from build123d import *

# Parameters (mm, degrees)
F0_R     = 1.45
F1_DEPTH = 1.5
F2_DEPTH = 18
F3_R     = 0.9
F4_DEPTH = 5
F6_DEPTH = 5
F7_R     = 3.8


with BuildPart() as f1:
    # F0 (on Top) → F1 (new body)
    with BuildSketch(Plane.XY):
        with BuildLine():
            Line((-2.6044162591, 5.2848328158), (-11.2348561883, 5.2848328158))
            Line((-11.2348561883, 5.2848328158), (-11.2348561883, -6.4651671842))
            Line((-11.2348561883, -6.4651671842), (-2.6044162591, -6.4651671842))
            ThreePointArc((-2.6044162591, -6.4651671842), (-0.1771907831, -2.6229563548), (3.2651438117, -5.5901671842))
            ThreePointArc((3.2651438117, -5.5901671842), (3.2323546411, -6.032501779), (3.1347038825, -6.4651671842))
            Line((3.1347038825, -6.4651671842), (7.3955837409, -6.4651671842))
            ThreePointArc((7.3955837409, -6.4651671842), (7.8542311215, -3.8048100771), (10.2651438117, -2.5901671842))
            Line((10.2651438117, -2.5901671842), (10.2651438117, 1.4098328158))
            ThreePointArc((10.2651438117, 1.4098328158), (7.8542311215, 2.6244757087), (7.3955837409, 5.2848328158))
            Line((7.3955837409, 5.2848328158), (3.1347038825, 5.2848328158))
            ThreePointArc((3.1347038825, 5.2848328158), (3.2323546411, 4.8521674106), (3.2651438117, 4.4098328158))
            ThreePointArc((3.2651438117, 4.4098328158), (-0.1771907831, 1.4426219864), (-2.6044162591, 5.2848328158))
        make_face()
        with Locations((-4.7348561883, -0.5901671842)):
            Circle(F0_R, mode=Mode.SUBTRACT)
        with Locations((5.2651438117, -0.5901671842)):
            Circle(F0_R, mode=Mode.SUBTRACT)
        with BuildLine():
            ThreePointArc((10.2651438117, -2.5901671842), (7.8542311215, -3.8048100771), (7.3955837409, -6.4651671842))
            Line((7.3955837409, -6.4651671842), (9.1089107037, -6.4651671842))
            ThreePointArc((9.1089107037, -6.4651671842), (8.9668275944, -4.9445086057), (10.2651438117, -4.1401671842))
            Line((10.2651438117, -4.1401671842), (10.2651438117, -2.5901671842))
        make_face()
        with BuildLine():
            Line((9.1089107037, 5.2848328158), (7.3955837409, 5.2848328158))
            ThreePointArc((7.3955837409, 5.2848328158), (7.8542311215, 2.6244757087), (10.2651438117, 1.4098328158))
            Line((10.2651438117, 1.4098328158), (10.2651438117, 2.9598328158))
            ThreePointArc((10.2651438117, 2.9598328158), (8.9668275944, 3.7641742373), (9.1089107037, 5.2848328158))
        make_face()
        with BuildLine():
            Line((9.1089107037, -6.4651671842), (7.3955837409, -6.4651671842))
            ThreePointArc((7.3955837409, -6.4651671842), (10.7074784065, -8.5573780136), (13.2651438117, -5.5901671842))
            ThreePointArc((13.2651438117, -5.5901671842), (12.6209876096, -3.7327496221), (10.9651438117, -2.672976755))
            ThreePointArc((10.9651438117, -2.672976755), (10.6175843829, -2.6109415057), (10.2651438117, -2.5901671842))
            Line((10.2651438117, -2.5901671842), (10.2651438117, -4.1401671842))
            ThreePointArc((10.2651438117, -4.1401671842), (11.2904486444, -4.5648623515), (11.7151438117, -5.5901671842))
            ThreePointArc((11.7151438117, -5.5901671842), (10.7266424539, -6.9647649448), (9.1089107037, -6.4651671842))
        make_face()
        with BuildLine():
            ThreePointArc((3.1347038825, 5.2848328158), (0.2651438117, 7.4098328158), (-2.6044162591, 5.2848328158))
            Line((-2.6044162591, 5.2848328158), (-0.8910892963, 5.2848328158))
            ThreePointArc((-0.8910892963, 5.2848328158), (0.2651438117, 5.8598328158), (1.4213769197, 5.2848328158))
            Line((1.4213769197, 5.2848328158), (3.1347038825, 5.2848328158))
        make_face()
        with BuildLine():
            Line((-0.8910892963, 5.2848328158), (-2.6044162591, 5.2848328158))
            ThreePointArc((-2.6044162591, 5.2848328158), (-0.1771907831, 1.4426219864), (3.2651438117, 4.4098328158))
            ThreePointArc((3.2651438117, 4.4098328158), (3.2323546411, 4.8521674106), (3.1347038825, 5.2848328158))
            Line((3.1347038825, 5.2848328158), (1.4213769197, 5.2848328158))
            ThreePointArc((1.4213769197, 5.2848328158), (1.6397415722, 4.8713314579), (1.7151438117, 4.4098328158))
            ThreePointArc((1.7151438117, 4.4098328158), (-0.1963548305, 3.0352350552), (-0.8910892963, 5.2848328158))
        make_face()
        with BuildLine():
            ThreePointArc((13.2651438117, 4.4098328158), (10.7074784065, 7.3770436452), (7.3955837409, 5.2848328158))
            Line((7.3955837409, 5.2848328158), (9.1089107037, 5.2848328158))
            ThreePointArc((9.1089107037, 5.2848328158), (10.7266424539, 5.7844305763), (11.7151438117, 4.4098328158))
            ThreePointArc((11.7151438117, 4.4098328158), (11.2904486444, 3.3845279831), (10.2651438117, 2.9598328158))
            Line((10.2651438117, 2.9598328158), (10.2651438117, 1.4098328158))
            ThreePointArc((10.2651438117, 1.4098328158), (10.6175843829, 1.4306071372), (10.9651438117, 1.4926423866))
            ThreePointArc((10.9651438117, 1.4926423866), (12.6209876096, 2.5524152537), (13.2651438117, 4.4098328158))
        make_face()
        with BuildLine():
            ThreePointArc((3.2651438117, -5.5901671842), (-0.1771907831, -2.6229563548), (-2.6044162591, -6.4651671842))
            Line((-2.6044162591, -6.4651671842), (-0.8910892963, -6.4651671842))
            ThreePointArc((-0.8910892963, -6.4651671842), (-0.1963548305, -4.2155694237), (1.7151438117, -5.5901671842))
            ThreePointArc((1.7151438117, -5.5901671842), (1.6397415722, -6.0516658264), (1.4213769197, -6.4651671842))
            Line((1.4213769197, -6.4651671842), (3.1347038825, -6.4651671842))
            ThreePointArc((3.1347038825, -6.4651671842), (3.2323546411, -6.032501779), (3.2651438117, -5.5901671842))
        make_face()
        with BuildLine():
            Line((-0.8910892963, -6.4651671842), (-2.6044162591, -6.4651671842))
            ThreePointArc((-2.6044162591, -6.4651671842), (0.2651438117, -8.5901671842), (3.1347038825, -6.4651671842))
            Line((3.1347038825, -6.4651671842), (1.4213769197, -6.4651671842))
            ThreePointArc((1.4213769197, -6.4651671842), (0.2651438117, -7.0401671842), (-0.8910892963, -6.4651671842))
        make_face()
        with BuildLine():
            ThreePointArc((10.9651438117, 1.4926423866), (10.6175843829, 1.4306071372), (10.2651438117, 1.4098328158))
            Line((10.2651438117, 1.4098328158), (10.2651438117, -2.5901671842))
            ThreePointArc((10.2651438117, -2.5901671842), (10.6175843829, -2.6109415057), (10.9651438117, -2.672976755))
            Line((10.9651438117, -2.672976755), (10.9651438117, 1.4926423866))
        make_face()
    extrude(amount=F1_DEPTH)

    # F0 (on Top) → F2 (join)
    with BuildSketch(Plane.XY):
        Polygon((11.6651438117, 8.2848328158), (-12.6348561883, 8.2848328158), (-12.6348561883, -9.4651671842), (14.7651438117, -9.4651671842), (14.7651438117, 8.2848328158), align=None)
        with BuildLine():
            Line((-11.2348561883, -6.4651671842), (-11.2348561883, 5.2848328158))
            Line((-11.2348561883, 5.2848328158), (-2.6044162591, 5.2848328158))
            ThreePointArc((-2.6044162591, 5.2848328158), (0.2651438117, 7.4098328158), (3.1347038825, 5.2848328158))
            Line((3.1347038825, 5.2848328158), (7.3955837409, 5.2848328158))
            ThreePointArc((7.3955837409, 5.2848328158), (10.7074784065, 7.3770436452), (13.2651438117, 4.4098328158))
            ThreePointArc((13.2651438117, 4.4098328158), (12.6209876096, 2.5524152537), (10.9651438117, 1.4926423866))
            Line((10.9651438117, 1.4926423866), (10.9651438117, -2.672976755))
            ThreePointArc((10.9651438117, -2.672976755), (12.6209876096, -3.7327496221), (13.2651438117, -5.5901671842))
            ThreePointArc((13.2651438117, -5.5901671842), (10.7074784065, -8.5573780136), (7.3955837409, -6.4651671842))
            Line((7.3955837409, -6.4651671842), (3.1347038825, -6.4651671842))
            ThreePointArc((3.1347038825, -6.4651671842), (0.2651438117, -8.5901671842), (-2.6044162591, -6.4651671842))
            Line((-2.6044162591, -6.4651671842), (-11.2348561883, -6.4651671842))
        make_face(mode=Mode.SUBTRACT)
    extrude(amount=F2_DEPTH)

    # F3 (on face) → F4 (cut)
    with BuildSketch(Plane.XY.offset(18)):
        with Locations((12.8651438117, -0.5901671842)):
            Circle(F3_R)
    extrude(amount=-F4_DEPTH, mode=Mode.SUBTRACT)

    # F5 (on face) → F6 (cut)
    with BuildSketch(Plane.YZ.offset(14.7651438117)):
        Polygon((-2.5901671842, 4.5), (-2.5901671842, 6), (0.0359741347, 6), (-0.6785203239, 7.7283125886), (-4.924895537, 18), (-8.171145565, 18), align=None)
        Polygon((0.0359741347, 6), (-2.5901671842, 6), (-2.5901671842, 4.5), (1.4098328158, 4.5), (1.4098328158, 6), align=None)
        with BuildLine():
            Line((-0.6785203239, 7.7283125886), (0.0359741347, 6))
            Line((0.0359741347, 6), (1.4098328158, 6))
            ThreePointArc((1.4098328158, 6), (0.5488853545, 7.0855555288), (-0.6785203239, 7.7283125886))
        make_face()
    extrude(amount=-F6_DEPTH, mode=Mode.SUBTRACT)

    # F7
    f7_edges = [f1.edges().sort_by_distance(p)[0] for p in [
        (14.765144, 8.284833, 9),
        (-12.634856, 8.284833, 9),
        (-12.634856, -9.465167, 9),
        (14.765144, -9.465167, 9),
    ]]
    fillet(f7_edges, radius=F7_R)


solid = f1.part
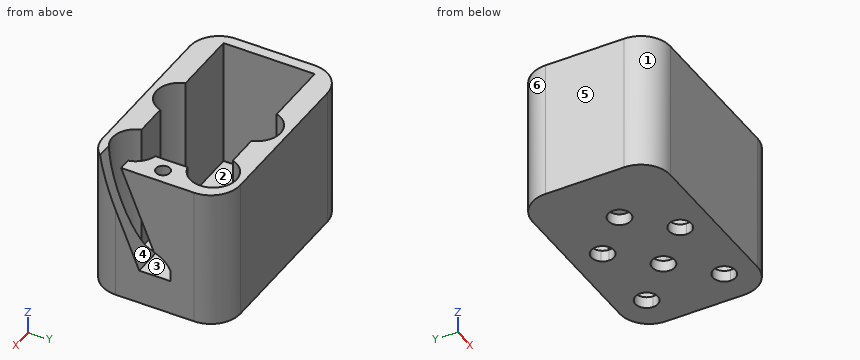
Check sheet for the modelled part. Datum: model origin and axes. Units: mm. Face numbers are marked on the shaded views. A direction names the side the tool comes from. Give positions to 0.01 mm unless a question says otherwise; leave off trailing zeros. Loops run counter-clockwise (first coordinate to the right, second up) from the corner with the lowest first, then second, coordinate; pieces in that order, holes last. Notation, with made-up numbers: M -37.75,18.25 L -8.75,18.25 A19 cw -8.75,26.25 Z; hole C 15,-37.75 d8. An arc over 180 degrees is marked long. Answer as a JSON object with one key per item and string values. Group by question number.
Q1. Cross-section at D-D on y = -7.75. Record the cut outline in (x, z).
Q2. Go/stop test with flat-tipped pins: P1, Ø1, axis at y = 6, z = 9, coming from the +X side; P2, Ø4, axis at x = 5.27, y = -0.59, coming from the -Z side; P3, Ø1.6, axis at x = 12.87, y = -0.59, coming from the +Z side; P4, Ø3.5, axis at x = 10.27, y = 4.41, coming from the +Z side. Record where each tip stops, or that it passes through.
Q3. Material ranges on line 1 along Y through (x, z) = (-7, 6.25); line 2 along Y through (x, z) = (11.25, 2); line 3 along X through (y, z) = (-3.5, 10), recorded low to high. Write a range as [from, to].
Q4. Access from +Z, -Z, +X, -X, +Y, -Y to the whole of each face (thin tool, end or side, straight path). Record for the marked faces 1, 2 and 3.
Q5. Cross-section at C-C on x = 5.25. Record the cut outline in (y, z).
Q6. Cross-section at A-A on z = 2. Record the cut outline in (x, y).
Q7. Release check for a two-part mould opening along Y. For the marked faces 4, 5 and 6 record: released by +Y, released by -Y, zero draft, split by the parting line, or undercut.
Q8. Cross-section at B-B on x = -7.25. Record the cut outline in (y, z).
Evaluation:
{
 "1": {"outline": "M -12.01,0 L 14.14,0 L 14.14,16.98 L 12.35,16.98 L 12.35,1.5 L 8.18,1.5 L 8.18,18 L 2.35,18 L 2.35,1.5 L -1.82,1.5 L -1.82,18 L -12.01,18 Z"},
 "2": {"P1": "stops at x = 14.63", "P2": "stops at z = 0", "P3": "stops at z = 13", "P4": "stops at z = 1.5"},
 "3": {"line 1": "y = [-9.47, -6.47], [5.28, 8.28]", "line 2": "y = [-9.45, -8.42], [-2.76, 1.58], [7.24, 8.27]", "line 3": "x = [-12.63, -11.23]"},
 "4": {"face 1": "+Z, -Z, -X, -Y", "face 2": "+Z", "face 3": "+X"},
 "5": {"outline": "M -9.47,0 L -2.04,0 L -2.04,1.5 L -6.47,1.5 L -6.47,18 L -9.47,18 Z; M 0.86,0 L 8.28,0 L 8.28,18 L 5.28,18 L 5.28,1.5 L 0.86,1.5 Z"},
 "6": {"outline": "M -12.63,-5.67 A3.8 ccw -8.83,-9.47 L 10.97,-9.47 A3.8 ccw 14.77,-5.67 L 14.77,4.48 A3.8 ccw 10.97,8.28 L -8.83,8.28 A3.8 ccw -12.63,4.48 Z; hole M -11.23,-6.47 L -2.6,-6.47 A3 ccw 3.13,-6.47 L 7.4,-6.47 A3 ccw long 10.97,-2.67 L 10.97,1.49 A3 ccw long 7.4,5.28 L 3.13,5.28 A3 ccw -2.6,5.28 L -11.23,5.28 Z"},
 "7": {"face 4": "undercut", "face 5": "zero draft", "face 6": "released by +Y"},
 "8": {"outline": "M -9.47,0 L 8.28,0 L 8.28,18 L 5.28,18 L 5.28,1.5 L -6.47,1.5 L -6.47,18 L -9.47,18 Z"}
}
